from build123d import *

# Parameters (mm, degrees)
F1_DEPTH = 55.88
F2_R     = 9.652
F3_DEPTH = 12.446
F4_W     = 57.15
F4_H     = 55.88
F5_DEPTH = 1.27


with BuildPart() as f1:
    # F0 (on Front) → F1 (new body)
    with BuildSketch(Plane.XZ):
        with BuildLine():
            Line((-33.601068, 0), (32.692932, 0))
            ThreePointArc((32.692932, 0), (-0.454068, 20.322772), (-33.601068, 0))
        make_face()
    extrude(amount=F1_DEPTH)

    # F2 (on face) → F3 (cut)
    with BuildSketch(Plane(origin=(0, 0, 0), x_dir=(1, 0, 0), z_dir=(0, 0, -1))):
        with Locations((0, 27.94)):
            Circle(F2_R)
    extrude(amount=-F3_DEPTH, mode=Mode.SUBTRACT)

    # F4 (on face) → F5 (cut)
    with BuildSketch(Plane(origin=(0, 0, 0), x_dir=(1, 0, 0), z_dir=(0, 0, -1))):
        with Locations((-0.454068, 27.94)):
            Rectangle(F4_W, F4_H)
    extrude(amount=-F5_DEPTH, mode=Mode.SUBTRACT)


solid = f1.part
CAD build for the part. Positions are in the model's coordinates, mm. A direction names the side the tool comes from. Give positions to 0.01 mm unless a question says otherwise; leave off trailing zeros. Write each loop counter-clockwise with the first axis right and the second up, starting at its lowest first coordinate (ties: lowest second). Pieces come first, ordered by that corner, then holes. Notation, with made-up numbers: M 9,-37 L 45,-37 A11 cw 45,-19 Z; hole C 38,-28 d6. An arc over 180 degrees is marked long. Put each result on its own line as item: value. Start each with the question number.
(1) Band-saw the part on D-D, the plane z = 6. Write the cut outline in (x, y), and give its area (3 significant figures).
(2) Mould opens along Y. For faces 4 (the face through (0, -28, 12.446)), 5 (the face through (-1, 0, 8)), 6 (the face through (0.12, -27.55, 20.32)) say: +Y half, -Y half, draft (parallel to the pull), parting line (faces both ways), or undercut.
(3) Probe L1, parallel to Y at x = 0, z = 5.5; L2, parallel to X at y = -27.94, z = 8; L3, parallel to X at y = -27.94, z = 7.5. List the from-to ranges inside material, lowest first.
(4) Band-saw the part on A-A, the plane y = -27.94. Write the cut outline in (x, z).
(5) Band-saw the part on B-B, the plane x = 0. Write the cut outline in (y, z), and give its area (3 significant figures).
(6) Band-saw the part on C-C, the plane z = 10.5. Write the cut outline in (x, y).
(7) Flat gauge pins, fed straight in: pin 1 Ø12 at (x, y) = (-2, -9.5) entering from -Z; pin 2 Ø6 at (x, y) = (-0.5, -26.5) entering from -Z; pin 3 Ø4 at (y, z) = (-6, 14.5) entering from +X. Where does each tip first touch, or does it go through?
(8) Which spindle directions (+Z, -Z, +X, -X, +Y, -Y) get a long thin tool onto all of the face, cutting with end or side? Do faces 1 (the face through (-7.66, -22.07, 6.78)), 2 (the face through (-31, -28, 0)), 3 (the face through (-7, -35, 1.27)). Say none if no direction does.
Response values:
1. outline: M -29.78,-55.88 L 28.88,-55.88 L 28.88,0 L -29.78,0 Z; hole C 0,-27.94 d19.3
1. area: 2,990 mm2
2. face 4: undercut
2. face 5: +Y half
2. face 6: draft
3. L1: y = -55.88 to -37.59, -18.29 to 0
3. L2: x = -28.11 to -9.65, 9.65 to 27.2
3. L3: x = -28.55 to -9.65, 9.65 to 27.64
4. outline: M -33.6,0 L -29.03,0 L -29.03,1.27 L -9.65,1.27 L -9.65,12.45 L 9.65,12.45 L 9.65,1.27 L 28.12,1.27 L 28.12,0 L 32.69,0 A37.19 ccw Z
5. outline: M -55.88,1.27 L -37.59,1.27 L -37.59,12.45 L -18.29,12.45 L -18.29,1.27 L 0,1.27 L 0,20.32 L -55.88,20.32 Z
5. area: 849 mm2
6. outline: M -25.64,-55.88 L 24.73,-55.88 L 24.73,0 L -25.64,0 Z; hole C 0,-27.94 d19.3
7. pin 1: stops at z = 1.27
7. pin 2: stops at z = 12.45
7. pin 3: stops at x = 22.37
8. face 1: -Z
8. face 2: -Z, +X, -X, +Y, -Y
8. face 3: -Z, +Y, -Y
